from build123d import *

# Parameters (mm, degrees)
F2_DEPTH = 12.7
F3_DEPTH = 12.192
F4_R     = 1.27
F5_DEPTH = 38.23583
F6_R     = 3.175
F7_DEPTH = 38.23239


with BuildPart() as f2:
    # F0 (on Right) → F2 (new body)
    with BuildSketch(Plane.YZ):
        Polygon((13.97679, 10.59016), (-49.52321, 10.59016), (-49.52321, -14.80984), (13.97679, -14.80984), (20.706118, -56.049787), (54.080267, -56.049787), (58.759574, -55.764545), (52.07679, -14.80984), (52.07679, 10.59016), (52.07679, 35.99016), (13.97679, 35.99016), align=None)
    extrude(amount=F2_DEPTH)

    # F1 (on Right) → F3 (cut)
    with BuildSketch(Plane.YZ):
        Polygon((16.135918, -12.26984), (22.865247, -53.509787), (54.002922, -53.509787), (55.800184, -53.400229), (49.53679, -15.01571), (49.53679, 10.59016), (49.53679, 33.45016), (16.51679, 33.45016), (16.51679, 8.05016), (-46.98321, 8.05016), (-46.98321, -12.26984), align=None)
    extrude(amount=F3_DEPTH, mode=Mode.SUBTRACT)

    # F4 (on face) → F5 (cut)
    with BuildSketch(Plane.XZ.offset(-13.97679)):
        with Locations((6.35, 15.67016)):
            Circle(F4_R)
    extrude(amount=-F5_DEPTH, mode=Mode.SUBTRACT)

    # F6 (on face) → F7 (cut)
    with BuildSketch(Plane.XZ.offset(-13.97679)):
        with Locations((6.35, 21.51216)):
            Circle(F6_R)
    extrude(amount=-F7_DEPTH, mode=Mode.SUBTRACT)


solid = f2.part
Part model, mm, in its own coordinate system. A direction names the side the tool comes from. Give positions to 0.01 mm unless a question says otherwise; leave off trailing zeros. Write each loop counter-clockwise with the first axis right and the second up, starting at its lowest first coordinate (ties: lowest second). Pieces come first, ordered by that corner, then holes.
1) Cut at A-A on z = 29. Write the cut outline in (x, y).
Resolved:
outline: (0, 13.98) - (12.7, 13.98) - (12.7, 52.08) - (0, 52.08) - (0, 49.54) - (12.19, 49.54) - (12.19, 16.52) - (0, 16.52) - close
2) Cut at C-C on x = 6.35. State how many separate pieces and enclosed holes the cut face has, then the cut area to 3 significant figures.
Resolved:
separate pieces: 4
enclosed holes: 0
area: 914 mm2
3) Cut at B-B on y = 43.5. Write the cut outline in (x, z).
Resolved:
outline: (0, -56.05) - (12.7, -56.05) - (12.7, 35.99) - (0, 35.99) - (0, 33.45) - (12.19, 33.45) - (12.19, -53.51) - (0, -53.51) - close
4) Which spindle directions (+Z, -Z, +X, -X, +Y, -Y) get a long thin tool onto all of the face, cutting with end or side? Do faces 5 (the face through (6, 49.537, 9)), 6 (the face through (5.662, 15.229, 18.413)), 7 (the face through (6, 13.977, 26)). Say none if no direction does.
Resolved:
face 5: -X
face 6: +Y, -Y
face 7: +Z, +X, -X, -Y
5) Two-plate mould, pull along Z, no slides. Class faces 1 (the face through (6.011, 52.712, -34.477)), 2 (the face through (6, 52.077, 10)), 3 (the face through (6.18, 50.79, 16.93)), 4 (the face through (6, -18, -14.81)): released by +Z, released by -Z, zero draft, split by the parting line, or undercut.
Resolved:
face 1: undercut
face 2: zero draft
face 3: undercut
face 4: released by -Z
6) Pin check, flat tips, straight feed: pin 1 (5 mm diameter, centred on x = 8.5, z = 16, fed in from +Y); pin 2 (7.5 mm diameter, centred on x = 6.35, z = 21.51, fed in from -Y); pin 3 (1.5 mm diameter, centred on x = 3.5, y = -31, fed in from +Z); pin 4 (4 mm diameter, centred on x = 6.35, z = 21.51, fed in from +Y). Stop position of each tip, or through.
Resolved:
pin 1: stops at y = 52.08
pin 2: stops at y = 13.98
pin 3: stops at z = 10.59
pin 4: passes through
7) Probe L1, parallel to Z at x = 10.25, y = -36; L2, parallel to Z at x = 6.75, y = 38; L3, parallel to Y at x = 8.25, z = 14. List the from-to ranges inside material, lowest first.
Resolved:
L1: z = -14.81 to -12.27, 8.05 to 10.59
L2: z = -56.05 to -53.51, 33.45 to 35.99
L3: y = 13.98 to 16.52, 49.54 to 52.08
